The figure shows three views and two pictorial views of one solid part (mm, origin at its lowest corner). Answer the questions. Give positions to 0.01 mm unless a question says otherwise; leave off trailing zeros. Write each loop counter-clockwise with the first axis right and the second up, starting at its lowest first coordinate (ties: lowest second). Pieces come first, ordered by that corner, then holes. Notation, with made-up numbers: M 75,70.5 L 101,70.5 A24 cw 101,94.5 Z; hole C -33.5,2 d5. An arc over 180 degrees is marked long. Return JSON: item names as keys, results as strings.
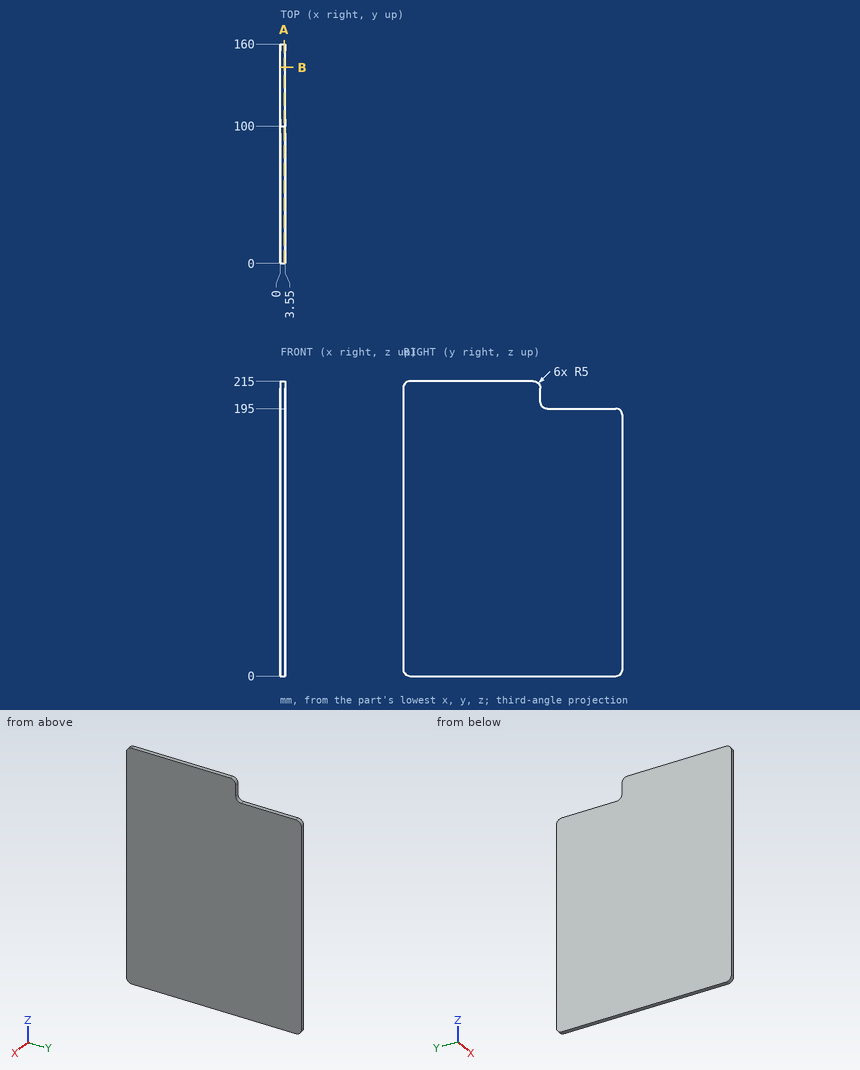
Item 1: A cutting plane is placed at B-B, the plane y = 143. Write down the section's boundary in (x, z), plus the area to 3 significant figures.
Geometry results:
{"outline": "M 0,0 L 3.55,0 L 3.55,195 L 0,195 Z", "area": "692 mm2"}
Item 2: Find the intervals of material crossed by line 1 (Z direction, x = 2.45, y = 133), in increasing order.
Geometry results:
{"line 1": "z = 0 to 195"}
Item 3: A cutting plane is placed at A-A, the plane x = 2.7. Write down the section's boundary in (y, z), plus the area to 3 significant figures.
Geometry results:
{"outline": "M 0,5 A5 ccw 5,0 L 155,0 A5 ccw 160,5 L 160,190 A5 ccw 155,195 L 105,195 A5 cw 100,200 L 100,210 A5 ccw 95,215 L 5,215 A5 ccw 0,210 Z", "area": "33,200 mm2"}
